from build123d import *

# Parameters (mm, degrees)
EXTRUDE_1_DEPTH     = 15
SKETCH_2_R          = 1.5
CUT_EXTRUDE_1_DEPTH = 37.523964735
SKETCH_3_R          = 2.425
CUT_EXTRUDE_2_DEPTH = 34.615472628


with BuildPart() as part:
    # 草图1 → 凸台-拉伸1 (new body)
    with BuildSketch(Plane.XY):
        Polygon((0, 0), (8, 0), (8, -25), (11, -25), (11, 3), (0, 3), (-11, 3), (-11, -25), (-8, -25), (-8, 0), align=None)
    extrude(amount=EXTRUDE_1_DEPTH)

    # 草图2 → 切除-拉伸1 (cut, through all)
    with BuildSketch(Plane(origin=(11, 0, 0), x_dir=(0, 0, -1), z_dir=(1, 0, 0))):
        with Locations((-7.5, -20)):
            Circle(SKETCH_2_R)
    extrude(amount=-CUT_EXTRUDE_1_DEPTH, mode=Mode.SUBTRACT)

    # 草图3 → 切除-拉伸2 (cut, through all)
    with BuildSketch(Plane(origin=(0, 3, 0), x_dir=(1, 0, 0), z_dir=(0, 1, 0))):
        with Locations(Location((0, -7.5, 0), (0, 0, 270))):
            Circle(SKETCH_3_R)
    extrude(amount=-CUT_EXTRUDE_2_DEPTH, mode=Mode.SUBTRACT)


solid = part.part
For this review, take the finished solid that the model builds, in its own axes (mm). A direction names the side the tool comes from. Give positions to 0.01 mm unless a question says otherwise; leave off trailing zeros. Loops run counter-clockwise (first coordinate to the right, second up) from the corner with the lowest first, then second, coordinate; pieces in that order, holes last.
Item 1: Take a section at A-A, the plane y = -20. State the section outline as (x, z) points.
Item 2: Take a section at C-C, the plane z = 7.5. State the section outline as (x, y) points (3 decimals), and give its area (3 significant figures).
Item 3: Take a section at D-D, the plane x = 9.5. State the section outline as (y, z) points.
Item 4: Draft analysis for pull direction Y (two halves, no side actions). For faces 1 (the flat face through (3, 3, 7)), 2 (the flat face through (-1.9, 0, 5.7)), 3 (the cylindrical face through (9.52, -18.99, 8.61)), state which applies: +Y half, -Y half, draft (parallel to the pull), parting line (faces both ways), or undercut.
Item 5: Tool access review of faces 4 (the flat face through (-8, -13, 7)), 5 (the flat face through (-8.2, -7.8, 15)): name each direction out of +Z, -Z, +X, -X, +Y, -Y from which nothing blocks a thin tool from reaching the whole face with its end or side.
Item 6: Insertion check: pin 1 (8 mm diameter, centred on x = 0, z = 7.5, fed in from +Y). The pin has a flat end and moves straight along its axis. Give the tip position at first contact, or say it passes through.
Item 7: Take a section at B-B, the plane x = 0. State the section outline as (y, z) points (3 decimals).
Item 8: For line 1 along X through (y, z) = (-12, 4.5); line 2 along Y through (x, z) = (9.85, 7.5); line 3 along X through (y, z) = (1.1, 7.5) (3 decimals), list the stretches that pass through material, from the lowest coordinate up.
Calculated:
1. outline: (-11, 0) - (-8, 0) - (-8, 6) - (-11, 6) - close; (-11, 9) - (-8, 9) - (-8, 15) - (-11, 15) - close; (8, 0) - (11, 0) - (11, 6) - (8, 6) - close; (8, 9) - (11, 9) - (11, 15) - (8, 15) - close
2. outline: (-11, -25) - (-8, -25) - (-8, -21.5) - (-11, -21.5) - close; (-11, -18.5) - (-8, -18.5) - (-8, 0) - (-2.425, 0) - (-2.425, 3) - (-11, 3) - close; (2.425, 0) - (8, 0) - (8, -18.5) - (11, -18.5) - (11, 3) - (2.425, 3) - close; (8, -25) - (11, -25) - (11, -21.5) - (8, -21.5) - close
2. area: 183 mm2
3. outline: (-25, 0) - (3, 0) - (3, 15) - (-25, 15) - close; hole circle Ø3 at (-20, 7.5)
4. face 1: +Y half
4. face 2: -Y half
4. face 3: undercut
5. face 4: +Z, -Z, -Y
5. face 5: +Z, +X, -X, +Y, -Y
6. pin 1: stops at y = 3
7. outline: (0, 0) - (3, 0) - (3, 5.075) - (0, 5.075) - close; (0, 9.925) - (3, 9.925) - (3, 15) - (0, 15) - close
8. line 1: x = -11 to -8, 8 to 11
8. line 2: y = -25 to -21.5, -18.5 to 3
8. line 3: x = -11 to -2.425, 2.425 to 11
